```python
from build123d import *

# Parameters (mm, degrees)
EXTRUDE_1_DEPTH     = 4.5
SKETCH_2_W          = 30
SKETCH_2_H          = 21
EXTRUDE_2_DEPTH     = 33
SKETCH_3_W          = 30
SKETCH_3_H          = 9
CUT_EXTRUDE_1_DEPTH = 33
SKETCH_4_R          = 7.5
CUT_EXTRUDE_2_DEPTH = 48.765049984
CUT_EXTRUDE_6_DEPTH = 48.765049984


with BuildPart() as part:
    # 草图1 → 凸台-拉伸1 (new body)
    with BuildSketch(Plane(origin=(0, 0, 0), x_dir=(1, 0, 0), z_dir=(0, 1, 0))):
        Polygon((-15, 13), (-13, 15), (13, 15), (15, 13), (15, -13), (13, -15), (-13, -15), (-15, -13), align=None)
    extrude(amount=EXTRUDE_1_DEPTH)

    # 草图2 → 凸台-拉伸2 (add)
    with BuildSketch(Plane(origin=(0, 4.5, 0), x_dir=(1, 0, 0), z_dir=(0, 1, 0))):
        Rectangle(SKETCH_2_W, SKETCH_2_H)
    extrude(amount=EXTRUDE_2_DEPTH)

    # 草图3 → 切除-拉伸1 (cut)
    with BuildSketch(Plane(origin=(0, 37.5, 0), x_dir=(1, 0, 0), z_dir=(0, 1, 0))):
        Rectangle(SKETCH_3_W, SKETCH_3_H)
    extrude(amount=-CUT_EXTRUDE_1_DEPTH, mode=Mode.SUBTRACT)

    # 草图4 → 切除-拉伸2 (cut, through all)
    with BuildSketch(Plane.XY.offset(10.5)):
        with Locations((0, 25.5)):
            Circle(SKETCH_4_R)
    extrude(amount=-CUT_EXTRUDE_2_DEPTH, mode=Mode.SUBTRACT)

    # 草图9 → 切除-拉伸6 (cut, through all)
    with BuildSketch(Plane.XY.offset(10.5)):
        Polygon((-15, 35.5), (-13, 37.5), (-15, 37.5), align=None)
        Polygon((13, 37.5), (15, 35.5), (15, 37.5), align=None)
    extrude(amount=-CUT_EXTRUDE_6_DEPTH, mode=Mode.SUBTRACT)


solid = part.part
```
CAD build for the part. Positions are in the model's coordinates, mm. A direction names the side the tool comes from. Coordinates: 2 decimals unless noted, no trailing zeros. Order: outer loops, then holes, each group sorted by start corner. A loop starts at its lowest first (then second) coordinate and runs counter-clockwise, first axis right, second up. Notation, with made-up numbers: (9.5, 88) - (23.5, 88) arc R27 ccw to (23.5, 115) - close; hole circle Ø5 at (53, -6.75). An arc over 180 degrees is marked (long way). Use a Markdown table: item, result. Add a question column.
(1) Saw through at B-B (x = 0). Give the cut face in (y, z), then the cut area to 3 significant figures.
(2) Saw through at A-A (y = 25.5). Give the cut face in (x, z).
(3) Saw through at C-C (y = 6.5). Give the cut face in (x, z), then the cut area to 3 significant figures.
(4) Flat gauge pins, fed straight in: pin 1 (1.3 mm diameter, centred on x = 5.5, z = 12.5, fed in from +Y); pin 2 (9 mm diameter, centred on x = 2.5, y = 21, fed in from -Z); pin 3 (4 mm diameter, centred on x = 9, y = 33.5, fed in from +Z). Where does each tip first touch, or does it go through?
(5) Which spindle directions (+Z, -Z, +X, -X, +Y, -Y) get a long thin tool onto all of the face, cutting with end or side? Do faces 5 (the face through (-0.2, 17.6, -4.5)), 6 (the face through (15, 18, 6)), 7 (the face through (0, 4.5, -13)). Say none if no direction does.
(6) Saw through at D-D (y = 21). Give the cut face in (x, z).
(7) Pull direction X, two halves, no side cores. Call faces 1 (the face through (-0.976, 32.936, 7.542)), 2 (the face through (0, 4.5, 13)), 3 (the face through (-0.976, 32.936, -7.458)), 4 (the face through (14, 2, -14)): +X half, -X half, draft (parallel to the pull), parting line (faces both ways), or undercut.
(8) Drill centre lines: line 1 along Y through (x, z) = (0, 9.15); line 2 along Z through (x, y) = (-0.25, 17); line 3 along Y through (x, z) = (-8.75, -0.25). Where is each one in solid material? Low to high. Write a range as [from, to].
Solved:
| question | item | result |
|---|---|---|
| 1 | outline | (0, -15) - (4.5, -15) - (4.5, -10.5) - (18, -10.5) - (18, -4.5) - (4.5, -4.5) - (4.5, 4.5) - (18, 4.5) - (18, 10.5) - (4.5, 10.5) - (4.5, 15) - (0, 15) - close; (33, -10.5) - (37.5, -10.5) - (37.5, -4.5) - (33, -4.5) - close; (33, 4.5) - (37.5, 4.5) - (37.5, 10.5) - (33, 10.5) - close |
| 1 | area | 351 mm² |
| 2 | outline | (-15, -10.5) - (-7.5, -10.5) - (-7.5, -4.5) - (-15, -4.5) - close; (-15, 4.5) - (-7.5, 4.5) - (-7.5, 10.5) - (-15, 10.5) - close; (7.5, -10.5) - (15, -10.5) - (15, -4.5) - (7.5, -4.5) - close; (7.5, 4.5) - (15, 4.5) - (15, 10.5) - (7.5, 10.5) - close |
| 3 | outline | (-15, -10.5) - (15, -10.5) - (15, -4.5) - (-15, -4.5) - close; (-15, 4.5) - (15, 4.5) - (15, 10.5) - (-15, 10.5) - close |
| 3 | area | 360 mm² |
| 4 | pin 1 | stops at y = 4.5 |
| 4 | pin 2 | stops at z = -10.5 |
| 4 | pin 3 | stops at z = 10.5 |
| 5 | face 5 | +X, -X, +Y |
| 5 | face 6 | +Z, -Z, +X, +Y, -Y |
| 5 | face 7 | -Z, +X, -X, +Y |
| 6 | outline | (-15, -10.5) - (-6, -10.5) - (-6, -4.5) - (-15, -4.5) - close; (-15, 4.5) - (-6, 4.5) - (-6, 10.5) - (-15, 10.5) - close; (6, -10.5) - (15, -10.5) - (15, -4.5) - (6, -4.5) - close; (6, 4.5) - (15, 4.5) - (15, 10.5) - (6, 10.5) - close |
| 7 | face 1 | undercut |
| 7 | face 2 | draft |
| 7 | face 3 | undercut |
| 7 | face 4 | +X half |
| 8 | line 1 | y = [0, 18], [33, 37.5] |
| 8 | line 2 | z = [-10.5, -4.5], [4.5, 10.5] |
| 8 | line 3 | y = [0, 4.5] |
